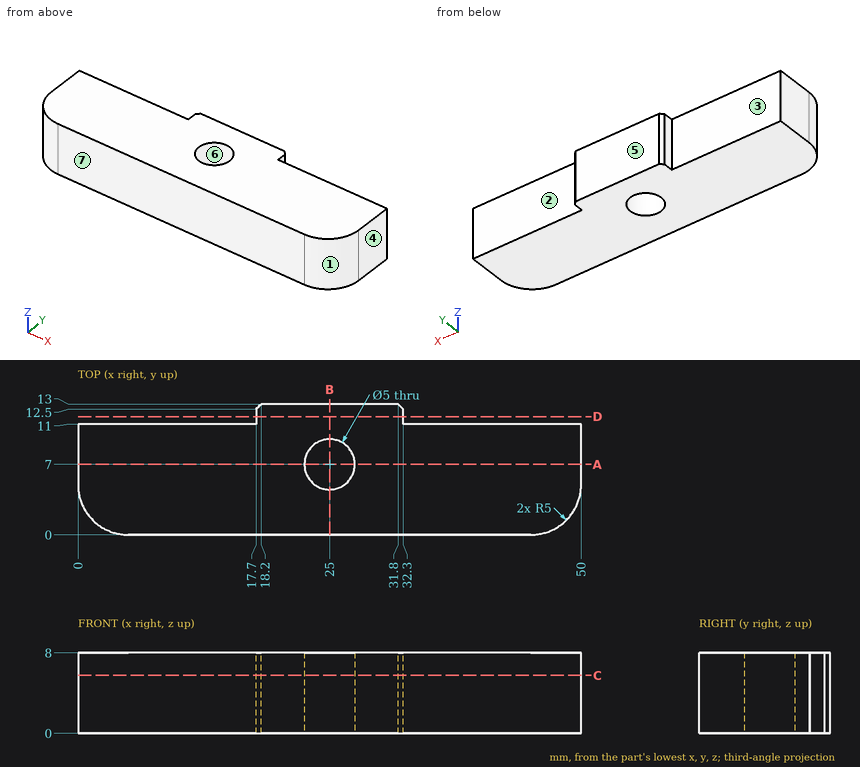
Check sheet for the drawn part. Datum: minimum x, y, z corner. Units: mm. A direction names the side the tool comes from. Give positions to 0.01 mm unless a question says otherwise; leave off trailing zeros. Order: outer loops, then holes, each group sorted by start corner. A loop starts at its lowest first (then second) coordinate and runs counter-clockwise, first axis right, second up. Notation, with made-up numbers: (-21.75, 73.5) -> (-1.75, 73.5) arc R24 cw to (-1.75, 110.5) -> close; hole circle Ø3 at (32.5, 83). An arc over 180 degrees is marked (long way). One line per item, written item: value.
(1) Scan lines: line 1 along Y through (x, z) = (25, 5.25); line 2 along X through (y, z) = (11.75, 0.75); line 3 along Y through (x, z) = (42, 7.25). Record each from-to range of solid material in increasing order. Write a range as [from, to].
Final values:
line 1: [0, 4.5], [9.5, 13]
line 2: [17.7, 32.3]
line 3: [0, 11]
(2) Sectioned sample at C-C on z = 5.75. Record the cut outline in (x, y), then the cut area to 3 significant figures.
Final values:
outline: (0, 5) arc R5 ccw to (5, 0) -> (45, 0) arc R5 ccw to (50, 5) -> (50, 11) -> (32.3, 11) -> (32.3, 12.5) -> (31.8, 13) -> (18.2, 13) -> (17.7, 12.5) -> (17.7, 11) -> (0, 11) -> close; hole circle Ø5 at (25, 7)
area: 549 mm^2
(3) Sectioned sample at A-A on y = 7. Record the cut outline in (x, z), then the cut area to 3 significant figures.
Final values:
outline: (0, 0) -> (22.5, 0) -> (22.5, 8) -> (0, 8) -> close; (27.5, 0) -> (50, 0) -> (50, 8) -> (27.5, 8) -> close
area: 360 mm^2
(4) Tool access check on the marked faces 1, 2 and 3. Record the directions out of +Z, -Z, +X, -X, +Y, -Y that give a thin tool (end or side, any length) a straight path to the whole face; none if there is none.
Final values:
face 1: +Z, -Z, +X, -Y
face 2: +Z, -Z, +X, +Y
face 3: +Z, -Z, -X, +Y
(5) Sectioned sample at D-D on y = 11.75. Record the cut outline in (x, z).
Final values:
outline: (17.7, 0) -> (32.3, 0) -> (32.3, 8) -> (17.7, 8) -> close
(6) Gauge pin test, flat ends, axial feed: pin 1 (1.2 mm diameter, centred on y = 11.5, z = 3.5, fed in from -X); pin 2 (0.8 mm diameter, centred on y = 11.5, z = 4, fed in from +X). Record the tip position at first contact, or that the pin passes through.
Final values:
pin 1: x = 0
pin 2: x = 32.3
(7) Draft check along Y on the marked faces 4, 5, 6 and 7. Enter one of: pulls with the +Y half, pulls with the -Y half, needs draft (parallel to the pull), parting line crosses it, or undercut.
Final values:
face 4: needs draft
face 5: pulls with the +Y half
face 6: undercut
face 7: pulls with the -Y half
(8) Sectioned sample at B-B on x = 25. Record the cut outline in (y, z).
Final values:
outline: (0, 0) -> (4.5, 0) -> (4.5, 8) -> (0, 8) -> close; (9.5, 0) -> (13, 0) -> (13, 8) -> (9.5, 8) -> close
